from build123d import *

# Parameters (mm, degrees)
SKETCH1_W                = 37
SKETCH1_H                = 27
SKETCH1_R                = 1.5
SKETCH1_R_2              = 6.3
BOSS_EXTRUDE2_DEPTH      = 3
BOSS_EXTRUDE4_DEPTH      = 27
BOSS_EXTRUDE4_DEPTH_BACK = 3
SKETCH2_W                = 37
SKETCH2_H                = 3
CUT_EXTRUDE1_DEPTH       = 55.753995288
CROQUIS1_W               = 9.332939374
CROQUIS1_H               = 27
SALIENTE_EXTRUIR1_DEPTH  = 10
CROQUIS2_W               = 9.332939374
CROQUIS2_H               = 27
CORTAR_EXTRUIR1_DEPTH    = 10
CROQUIS3_W               = 10.381853436
CROQUIS3_H               = 27
SALIENTE_EXTRUIR2_DEPTH  = 10
CROQUIS4_W               = 10.381853436
CROQUIS4_H               = 27
CORTAR_EXTRUIR3_DEPTH    = 10
CROQUIS5_W               = 9.124203914
CROQUIS5_H               = 27
SALIENTE_EXTRUIR3_DEPTH  = 10
CROQUIS6_W               = 9.124203914
CROQUIS6_H               = 27
CORTAR_EXTRUIR5_DEPTH    = 10


with BuildPart() as part:
    # Sketch1 → Boss-Extrude2 (new body)
    with BuildSketch(Plane.XY):
        with Locations((18.5, 16.5)):
            Rectangle(SKETCH1_W, SKETCH1_H)
        with Locations((10.75, 8.076606241)):
            Circle(SKETCH1_R, mode=Mode.SUBTRACT)
        with Locations((18.5, 14.5)):
            Circle(SKETCH1_R_2, mode=Mode.SUBTRACT)
        with Locations((26.25, 8.076606241)):
            Circle(SKETCH1_R, mode=Mode.SUBTRACT)
        with Locations((3, 21.5)):
            Circle(SKETCH1_R, mode=Mode.SUBTRACT)
        with Locations((34, 21.5)):
            Circle(SKETCH1_R, mode=Mode.SUBTRACT)
    extrude(amount=BOSS_EXTRUDE2_DEPTH)

    # Sketch2 → Boss-Extrude4 (add, two sides: drawn at the far end of the back side and taken through both)
    with BuildSketch(Plane.XY.offset(3).offset(-BOSS_EXTRUDE4_DEPTH_BACK)):
        with Locations((18.5, 1.5)):
            Rectangle(SKETCH2_W, SKETCH2_H)
    extrude(amount=BOSS_EXTRUDE4_DEPTH + BOSS_EXTRUDE4_DEPTH_BACK)

    # Sketch4 → Cut-Extrude1 (cut, through all)
    with BuildSketch(Plane(origin=(0, 3, 0), x_dir=(1, 0, 0), z_dir=(0, 1, 0))):
        with BuildLine():
            Line((5.5, -8.25), (9.5, -8.25))
            ThreePointArc((9.5, -8.25), (11, -9.75), (9.5, -11.25))
            Line((9.5, -11.25), (5.5, -11.25))
            ThreePointArc((5.5, -11.25), (4, -9.75), (5.5, -8.25))
        make_face()
        with BuildLine():
            Line((27.5, -8.25), (31.5, -8.25))
            ThreePointArc((31.5, -8.25), (33, -9.75), (31.5, -11.25))
            Line((31.5, -11.25), (27.5, -11.25))
            ThreePointArc((27.5, -11.25), (26, -9.75), (27.5, -8.25))
        make_face()
        with BuildLine():
            Line((27.5, -21.75), (31.5, -21.75))
            ThreePointArc((31.5, -21.75), (33, -23.25), (31.5, -24.75))
            Line((31.5, -24.75), (27.5, -24.75))
            ThreePointArc((27.5, -24.75), (26, -23.25), (27.5, -21.75))
        make_face()
        with BuildLine():
            Line((5.5, -21.75), (9.5, -21.75))
            ThreePointArc((9.5, -21.75), (11, -23.25), (9.5, -24.75))
            Line((9.5, -24.75), (5.5, -24.75))
            ThreePointArc((5.5, -24.75), (4, -23.25), (5.5, -21.75))
        make_face()
    extrude(amount=-CUT_EXTRUDE1_DEPTH, mode=Mode.SUBTRACT)

    # Croquis1 → Saliente-Extruir1 (add)
    with BuildSketch(Plane(origin=(0, 3, 0), x_dir=(1, 0, 0), z_dir=(0, 1, 0))):
        with Locations((26.333530313, -16.5)):
            Rectangle(CROQUIS1_W, CROQUIS1_H)
    extrude(amount=SALIENTE_EXTRUIR1_DEPTH)

    # Croquis2 → Cortar-Extruir1 (cut)
    with BuildSketch(Plane(origin=(0, 3, 0), x_dir=(1, 0, 0), z_dir=(0, 1, 0))):
        with Locations((26.333530313, -16.5)):
            Rectangle(CROQUIS2_W, CROQUIS2_H)
    extrude(amount=CORTAR_EXTRUIR1_DEPTH, mode=Mode.SUBTRACT)

    # Croquis3 → Saliente-Extruir2 (add)
    with BuildSketch(Plane(origin=(0, 3, 0), x_dir=(1, 0, 0), z_dir=(0, 1, 0))):
        with Locations((25.809073282, -16.5)):
            Rectangle(CROQUIS3_W, CROQUIS3_H)
    extrude(amount=SALIENTE_EXTRUIR2_DEPTH)

    # Croquis4 → Cortar-Extruir3 (cut)
    with BuildSketch(Plane(origin=(0, 3, 0), x_dir=(1, 0, 0), z_dir=(0, 1, 0))):
        with Locations((25.809073282, -16.5)):
            Rectangle(CROQUIS4_W, CROQUIS4_H)
    extrude(amount=CORTAR_EXTRUIR3_DEPTH, mode=Mode.SUBTRACT)

    # Croquis5 → Saliente-Extruir3 (add)
    with BuildSketch(Plane(origin=(0, 3, 0), x_dir=(1, 0, 0), z_dir=(0, 1, 0))):
        with Locations((26.437898043, -16.5)):
            Rectangle(CROQUIS5_W, CROQUIS5_H)
    extrude(amount=SALIENTE_EXTRUIR3_DEPTH)

    # Croquis6 → Cortar-Extruir5 (cut)
    with BuildSketch(Plane(origin=(0, 3, 0), x_dir=(1, 0, 0), z_dir=(0, 1, 0))):
        with Locations((26.437898043, -16.5)):
            Rectangle(CROQUIS6_W, CROQUIS6_H)
    extrude(amount=CORTAR_EXTRUIR5_DEPTH, mode=Mode.SUBTRACT)


solid = part.part
Model file for the job. Use its own axes, mm. A direction names the side the tool comes from. Give positions to 0.01 mm unless a question says otherwise; leave off trailing zeros. Write each loop counter-clockwise with the first axis right and the second up, starting at its lowest first coordinate (ties: lowest second). Pieces come first, ordered by that corner, then holes. Notation, with made-up numbers: (71, 52.5) -> (124, 52.5) arc R9 ccw to (124, 57.5) -> close; hole circle Ø7 at (1.5, 68.25). An arc over 180 degrees is marked (long way). Write item = value, one per line.
(1) Mould opens along X. For faces 4 (the face through (4, 1.5, 9.8)), 5 (the face through (0, 2.7, 8.3)), 6 (the face through (18, 30, 1)) say: released by +X, released by -X, zero draft, split by the parting line, or undercut.
Determined:
face_4 = undercut
face_5 = released by -X
face_6 = zero draft
(2) Tool access for faces 1 (the face through (29, 2, 21.75)), 2 (the face through (13.86, 18.76, 1.48)), 3 (the face through (18, 3, 16)): list every direction of +Z, -Z, +X, -X, +Y, -Y with a clear straight run to the whole face (end or side of a thin tool).
Determined:
face_1 = +Y, -Y
face_2 = +Z, -Z
face_3 = +Z, +X, -X, +Y
(3) Probe line 1 along X through (y, z) = (14.5, 1.65); line 2 along Y through (x, z) = (26.25, 1.35); line 3 along Z through (x, y) = (24.5, 20.25). List the from-to ranges inside material, lowest first.
Determined:
line_1 = 0 to 12.2, 24.8 to 37
line_2 = 0 to 6.58, 9.58 to 30
line_3 = 0 to 3
(4) Slice it at D-D, the plane y = 17. Give the cut face in (x, z), then the cut area to 3 significant figures.
Determined:
outline = (0, 0) -> (12.72, 0) -> (12.72, 3) -> (0, 3) -> close; (24.28, 0) -> (37, 0) -> (37, 3) -> (24.28, 3) -> close
area = 76.3 mm2
(5) Flat gauge pins, fed straight in: P1, Ø6, axis at y = 21, z = 8.5, coming from the -X side; P2, Ø1.5, axis at x = 29.5, z = 25, coming from the +Y side; P3, Ø8, axis at x = 20, y = 10.5, coming from the +Z side. Where does each tip first touch, or does it go through?
Determined:
P1 = through
P2 = 3
P3 = 3
(6) Slice it at C-C, the plane y = 2.25. Give the cut face in (x, z), then the cut area to 3 significant figures.
Determined:
outline = (0, 0) -> (37, 0) -> (37, 30) -> (0, 30) -> close; hole (5.5, 8.25) -> (9.5, 8.25) arc R1.5 ccw to (9.5, 11.25) -> (5.5, 11.25) arc R1.5 ccw to start; hole (5.5, 21.75) -> (9.5, 21.75) arc R1.5 ccw to (9.5, 24.75) -> (5.5, 24.75) arc R1.5 ccw to start; hole (27.5, 8.25) -> (31.5, 8.25) arc R1.5 ccw to (31.5, 11.25) -> (27.5, 11.25) arc R1.5 ccw to start; hole (27.5, 21.75) -> (31.5, 21.75) arc R1.5 ccw to (31.5, 24.75) -> (27.5, 24.75) arc R1.5 ccw to start
area = 1,030 mm2
(7) Slice it at A-A, the plane x = 34. Give the cut face in (y, z).
Determined:
outline = (0, 0) -> (20, 0) -> (20, 3) -> (3, 3) -> (3, 30) -> (0, 30) -> close; (23, 0) -> (30, 0) -> (30, 3) -> (23, 3) -> close
(8) Slice it at B-B, the plane z = 9.75. Give the cut face in (x, y).
Determined:
outline = (0, 0) -> (4, 0) -> (4, 3) -> (0, 3) -> close; (11, 0) -> (26, 0) -> (26, 3) -> (11, 3) -> close; (33, 0) -> (37, 0) -> (37, 3) -> (33, 3) -> close
